Design review of the part built by this model. Coordinates are the model's own, in mm. A direction names the side the tool comes from. Coordinates: 2 decimals unless noted, no trailing zeros. Loops run counter-clockwise (first coordinate to the right, second up) from the corner with the lowest first, then second, coordinate; pieces in that order, holes last. Notation, with made-up numbers: M -34.75,12.25 L -20.75,12.25 A31 ccw -20.75,37.25 Z; hole C 54.5,8.5 d9. An arc over 180 degrees is marked long. Put each result on its own line as item: value. Start each with the question number.
(1) Take a section at D-D, the plane x = 25. Give the boundary of the cut face in (y, z), then the cut area to 3 significant figures.
(2) Clearance check with flat-ended pins moving along their axes: pin 1 (17.5 mm diameter, centred on x = -6.5, z = 1.5, fed in from -Y); pin 2 (5 mm diameter, centred on x = 11.5, y = 16, fed in from -Z); pin 3 (6.5 mm diameter, centred on x = -7.73, z = 23.78, fed in from -Y); pin 4 (2 mm diameter, centred on y = 3.5, z = -19, fed in from +X). State where each tip first meets the part, or that it passes through.
(3) The part is to be moulded in two halves that separate along X. For faces 1 (the cylindrical face through (-12.865, 18.734, 17.63)), 2 (the cylindrical face through (-27.5, 43.3, -0.1)), 3 (the cylindrical face through (12.792, 18.734, 17.683)), say which applies: +X half, -X half, draft (parallel to the pull), parting line (faces both ways), or undercut.
(4) Take a section at C-C, the plane z = 0. Count the separate pieces of the cut face and the enclosed holes in it, then the cut area to 3 significant figures.
(5) For faces 4 (the cylindrical face through (17.794, -3.204, -14.112)), 5 (the cylindrical face through (6.1, 20.28, 19.05)), 6 (the cylindrical face through (-12.792, 18.734, -17.683)), list the 3-axis set-ups (+Z, -Z, +X, -X, +Y, -Y) from which the entire face can be reached by the end or side of a thin tool; tool diameter is ignored.
(6) Take a section at B-B, the plane y = 12.5. Give the boundary of the cut face in (x, z) (3 decimals).
(7) Take a section at A-A, the plane x = 0. Give the boundary of the cut face in (y, z) (3 decimals).
(8) For probe 1 along X at (y, z) = (15, 0); probe 2 along Y at (x, z) = (25, 13); probe 3 along X at (y, z) = (41, -26), list the stretches that pass through material, from the lowest coordinate up. Write a range as [from, to].
```python
from build123d import *

# Parameters (mm, degrees)
SKETCH2_R           = 21.825
SKETCH2_R_2         = 18.19
BOSS_EXTRUDE1_DEPTH = 40
SKETCH4_R           = 29.5
SKETCH4_R_2         = 18.19
BOSS_EXTRUDE3_DEPTH = 6.5
BOSS_EXTRUDE4_START = 6.5
SKETCH5_R           = 29
SKETCH5_R_2         = 18.19
BOSS_EXTRUDE4_DEPTH = 6.5
FILLET1_R           = 2
HOLE1_D             = 5
CIRPATTERN1_COUNT   = 10
SKETCH9_R           = 5
CUT_EXTRUDE1_DEPTH  = 40
CIRPATTERN2_COUNT   = 10


with BuildPart() as part:
    # Sketch2 → Boss-Extrude1 (new body)
    with BuildSketch(Plane(origin=(0, 0, 0), x_dir=(1, 0, 0), z_dir=(0, 1, 0))):
        with Locations(Location((0, 0, 0), (0, 0, 270))):
            Circle(SKETCH2_R)
        with Locations(Location((0, 0, 0), (0, 0, 270))):
            Circle(SKETCH2_R_2, mode=Mode.SUBTRACT)
    extrude(amount=BOSS_EXTRUDE1_DEPTH)

    # Sketch4 → Boss-Extrude3 (add)
    with BuildSketch(Plane(origin=(0, 40, 0), x_dir=(1, 0, 0), z_dir=(0, 1, 0))):
        with Locations(Location((0, 0, 0), (0, 0, 90))):
            Circle(SKETCH4_R)
        with Locations(Location((0, 0, 0), (0, 0, 270))):
            Circle(SKETCH4_R_2, mode=Mode.SUBTRACT)
    extrude(amount=BOSS_EXTRUDE3_DEPTH)

    # Sketch5 → Boss-Extrude4 (add)
    with BuildSketch(Plane.XZ.offset(BOSS_EXTRUDE4_START)):
        with Locations(Location((0, 0, 0), (0, 0, 90))):
            Circle(SKETCH5_R)
        with Locations(Location((0, 0, 0), (0, 0, 270))):
            Circle(SKETCH5_R_2, mode=Mode.SUBTRACT)
    extrude(amount=-BOSS_EXTRUDE4_DEPTH)

    # Fillet1
    fillet1_edges = [part.edges().sort_by_distance(p)[0] for p in [
        (0, 40, -21.825),
    ]]
    fillet(fillet1_edges, radius=FILLET1_R)

    # Hole1 (through all)
    with Locations(Plane(origin=(0, -6.5, 0), x_dir=(-1, 0, 0), z_dir=(0, -1, 0))):
        with Locations((25, 0)):
            hole1 = Hole(HOLE1_D / 2)

    # CirPattern1: Hole1 ×10 about axis
    cirpattern1_axis = Axis((0, 0, 0), (0, 1, 0))
    for i in range(1, CIRPATTERN1_COUNT):
        add(hole1.rotate(cirpattern1_axis, i * 360 / CIRPATTERN1_COUNT), mode=Mode.SUBTRACT)

    # Sketch9 → Cut-Extrude1 (cut)
    with BuildSketch(Plane.XZ.offset(-40)):
        with Locations((-20.225424859, 14.694631307)):
            Circle(SKETCH9_R)
    cut_extrude1 = extrude(amount=CUT_EXTRUDE1_DEPTH, mode=Mode.SUBTRACT)

    # CirPattern2: Cut-Extrude1 ×10 about axis
    cirpattern2_axis = Axis((0, 0, 0), (0, 1, 0))
    for i in range(1, CIRPATTERN2_COUNT):
        add(cut_extrude1.rotate(cirpattern2_axis, i * 360 / CIRPATTERN2_COUNT), mode=Mode.SUBTRACT)


solid = part.part
```
Computed values:
1. outline: M -6.5,-14.7 L 0,-14.7 L 0,-2.5 L -6.5,-2.5 Z; M -6.5,2.5 L 0,2.5 L 0,14.7 L -6.5,14.7 Z; M 40,-15.66 L 46.5,-15.66 L 46.5,-2.5 L 40,-2.5 Z; M 40,2.5 L 46.5,2.5 L 46.5,15.66 L 40,15.66 Z
1. area: 330 mm^2
2. pin 1: passes through
2. pin 2: stops at z = -19.36
2. pin 3: stops at y = -6.5
2. pin 4: stops at x = 12.34
3. face 1: -X half
3. face 2: undercut
3. face 3: +X half
4. separate pieces: 6
4. enclosed holes: 0
4. area: 302 mm^2
5. face 4: +Y, -Y
5. face 5: +Z
5. face 6: -Z, -X
6. outline: M -21.527,-3.597 A21.825 ccw -19.529,-9.743 A5 cw -15.301,-15.563 A21.825 ccw -10.073,-19.362 A5 cw -3.232,-21.584 A21.825 ccw 3.232,-21.584 A5 cw 10.073,-19.362 A21.825 ccw 15.301,-15.563 A5 cw 19.529,-9.743 A21.825 ccw 21.527,-3.597 A5 cw 21.527,3.597 A21.825 ccw 19.529,9.743 A5 cw 15.301,15.563 A21.825 ccw 10.073,19.362 A5 cw 3.232,21.584 A21.825 ccw -3.232,21.584 A5 cw -10.073,19.362 A21.825 ccw -15.301,15.563 A5 cw -19.529,9.743 A21.825 ccw -21.527,3.597 A5 cw Z; hole C 0,0 d36.38
7. outline: M -6.5,-29 L 0,-29 L 0,-21.825 L 38,-21.825 A2 cw 40,-23.825 L 40,-29.5 L 46.5,-29.5 L 46.5,-18.19 L -6.5,-18.19 Z; M -6.5,18.19 L 46.5,18.19 L 46.5,29.5 L 40,29.5 L 40,23.825 A2 cw 38,21.825 L 0,21.825 L 0,29 L -6.5,29 Z
8. probe 1: x = [-20, -18.19], [18.19, 20]
8. probe 2: y = [-6.5, 0], [40, 46.5]
8. probe 3: x = [-13.94, -8.87], [-6.58, 6.58], [8.87, 13.94]
